Geometry: final body of the model. Coordinates: model frame, mm. Face numbers are marked on the shaded views. Give positions to 0.01 mm unless a question says otherwise; leave off trailing zeros. Write each loop counter-clockwise with the first axis right and the second up, starting at its lowest first coordinate (ties: lowest second). Pieces come first, ordered by that corner, then holes. Notation, with made-up numbers: (12, -16.75) -> (70, -16.75) arc R10 ccw to (70, -9.75) -> close; hole circle Ø2 at (-25.5, 15). An arc over 180 degrees is marked (long way). Use CSV: the item, a comma, the result in double quotes. Start each with the question number.
1) Section A-A (y = 0). Output: boundary loops of the cut face in (x, z), plus the area to 3 significant figures.
2) Section D-D (z = 14.75). Output: boundary loops of the cut face in (x, y), plus the area to 3 significant figures.
3) Contact query for flat-ended pins moving along their axis: P1, Ø8, axis at x = 0, y = 0, coming from the +Z side; P2, Ø1, axis at x = 6.5, z = 11, coming from the -Y side; P3, Ø8, axis at y = 5, z = 14, coming from the +X side. Output: stop coordinate, or through.
4) Section C-C (z = 7). Output: boundary loops of the cut face in (x, y).
5) Draft query along X for the marked faces 1, 2 and 3. Return one class per face: pulls with the +X half, pulls with the -X half, needs draft (parallel to the pull), parting line crosses it, or undercut.
6) Material intervals for line 1 (Y direction, x = 0, z = 5.75); line 2 (Y direction, x = 0, z = 18.25); line 3 (Z direction, x = -0.5, y = -4.25), sorted ascending. Write a range as [from, to].
```python
from build123d import *

# Parameters (mm, degrees)
SKETCH_1_R          = 10
EXTRUDE_1_DEPTH     = 25
SKETCH_2_R          = 6
CUT_EXTRUDE_1_DEPTH = 12.5
SKETCH_3_R          = 3
CUT_EXTRUDE_2_DEPTH = 15
FILLET_1_R          = 0.5


with BuildPart() as part:
    # 草图1 → 凸台-拉伸1 (new body)
    with BuildSketch(Plane.XY):
        Circle(SKETCH_1_R)
    extrude(amount=EXTRUDE_1_DEPTH)

    # 草图2 → 切除-拉伸1 (cut)
    with BuildSketch(Plane.XY.offset(25)):
        Circle(SKETCH_2_R)
    extrude(amount=-CUT_EXTRUDE_1_DEPTH, mode=Mode.SUBTRACT)

    # 草图3 → 切除-拉伸2 (cut)
    with BuildSketch(Plane(origin=(0, 0, 0), x_dir=(-1, 0, 0), z_dir=(0, 0, -1))):
        Circle(SKETCH_3_R)
    extrude(amount=-CUT_EXTRUDE_2_DEPTH, mode=Mode.SUBTRACT)

    # 圆角1
    fillet_1_edges = [part.edges().sort_by_distance(p)[0] for p in [
        (3, 0, 0),
        (-10, 0, 0),
        (-10, 0, 25),
        (-6, 0, 25),
    ]]
    fillet(fillet_1_edges, radius=FILLET_1_R)


solid = part.part
```
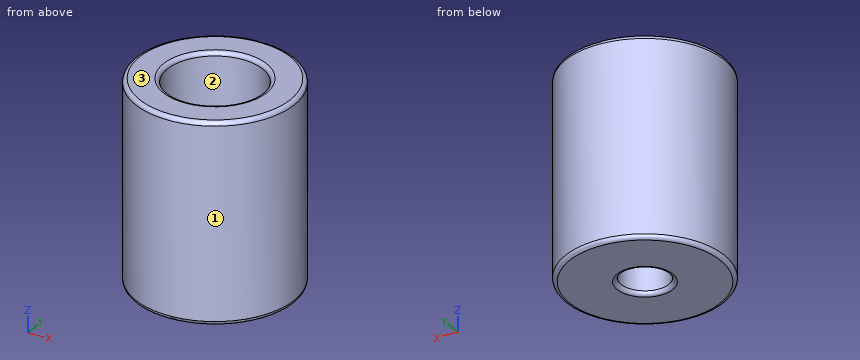
Answers follow:
1,outline,"(-10, 0.5) arc R0.5 ccw to (-9.5, 0) -> (-3.5, 0) arc R0.5 ccw to (-3, 0.5) -> (-3, 12.5) -> (-6, 12.5) -> (-6, 24.5) arc R0.5 ccw to (-6.5, 25) -> (-9.5, 25) arc R0.5 ccw to (-10, 24.5) -> close; (3, 0.5) arc R0.5 ccw to (3.5, 0) -> (9.5, 0) arc R0.5 ccw to (10, 0.5) -> (10, 24.5) arc R0.5 ccw to (9.5, 25) -> (6.5, 25) arc R0.5 ccw to (6, 24.5) -> (6, 12.5) -> (3, 12.5) -> close"
1,area,"275 mm^2"
2,outline,"circle Ø20 at (0, 0); hole circle Ø12 at (0, 0)"
2,area,"201 mm^2"
3,P1,"stops at z = 12.5"
3,P2,"stops at y = -8"
3,P3,"stops at x = 9.95"
4,outline,"circle Ø20 at (0, 0); hole circle Ø6 at (0, 0)"
5,face 1,"parting line crosses it"
5,face 2,"undercut"
5,face 3,"needs draft"
6,line 1,"y = [-10, -3], [3, 10]"
6,line 2,"y = [-10, -6], [6, 10]"
6,line 3,"z = [0, 12.5]"
